Input: dimensioned drawing with shaded views. Units: mm. Origin: part minimum x, y, z. Give positions to 0.01 mm unless a question says otherwise; leave off trailing zeros. Order: outer loops, then holes, each group sorted by start corner. A loop starts at its lowest first (then second) coordinate and runs counter-clockwise, first axis right, second up.
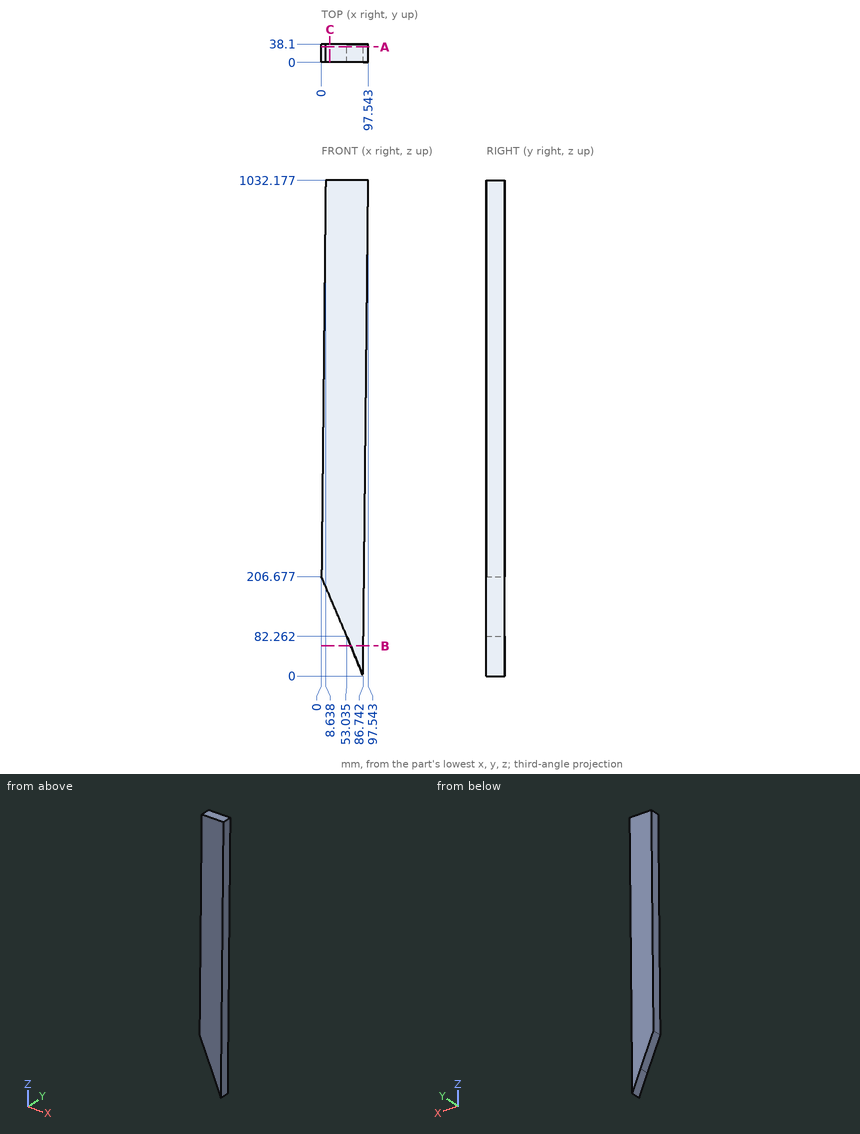
1) Pin query (flat end, axial travel): pin 1 (1 mm diameter, centred on x = 11, y = 22.5, fed in from -Z); pin 2 (4 mm diameter, centred on y = 33.5, z = 137, fed in from +X); pin 3 (2 mm diameter, centred on x = 51, y = 7.5, fed in from -Z). Return the tip coordinate at first contact, or that it passes through.
Report:
pin 1: stops at z = 179.7
pin 2: stops at x = 88.2
pin 3: stops at z = 84.69
2) Section query A-A, the plane y = 32. Return the cut outline in (x, z) (1 decimal).
Report:
outline: (0, 206.7) - (53, 82.3) - (86.7, 0) - (97.5, 1032.2) - (8.6, 1032.2) - close
3) Material intervals for L1, parallel to Z at x = 18.5, y = 14 (1 decimal); L2, parallel to X at y = 7.5, z = 820; L3, parallel to Z at x = 50.5, y = 17.5 (1 decimal), sorted ascending.
Report:
L1: z = 163.3 to 1032.2
L2: x = 6.42 to 95.32
L3: z = 88.2 to 1032.2
4) Section query B-B, the plane z = 62.5. Return the cut outline in (x, y), and give its area (3 significant figures).
Report:
outline: (61.13, 0) - (87.4, 0) - (87.4, 38.1) - (61.13, 38.1) - close
area: 1,000 mm2
5) Section query C-C, the plane x = 17.5. Return the cut outline in (y, z), and give its area (3 significant figures).
Report:
outline: (0, 165.62) - (38.1, 165.62) - (38.1, 1032.18) - (0, 1032.18) - close
area: 33,000 mm2
